Geometry: see drawing. Coordinates: mm, zero at the bounding-box minimum. A direction names the side the tool comes from. Coordinates: 2 decimals unless noted, no trailing zeros. Write each loop counter-clockwise with the first axis right and the second up, starting at its lowest first coordinate (ties: lowest second). Pieces come first, ordered by that corner, then holes.
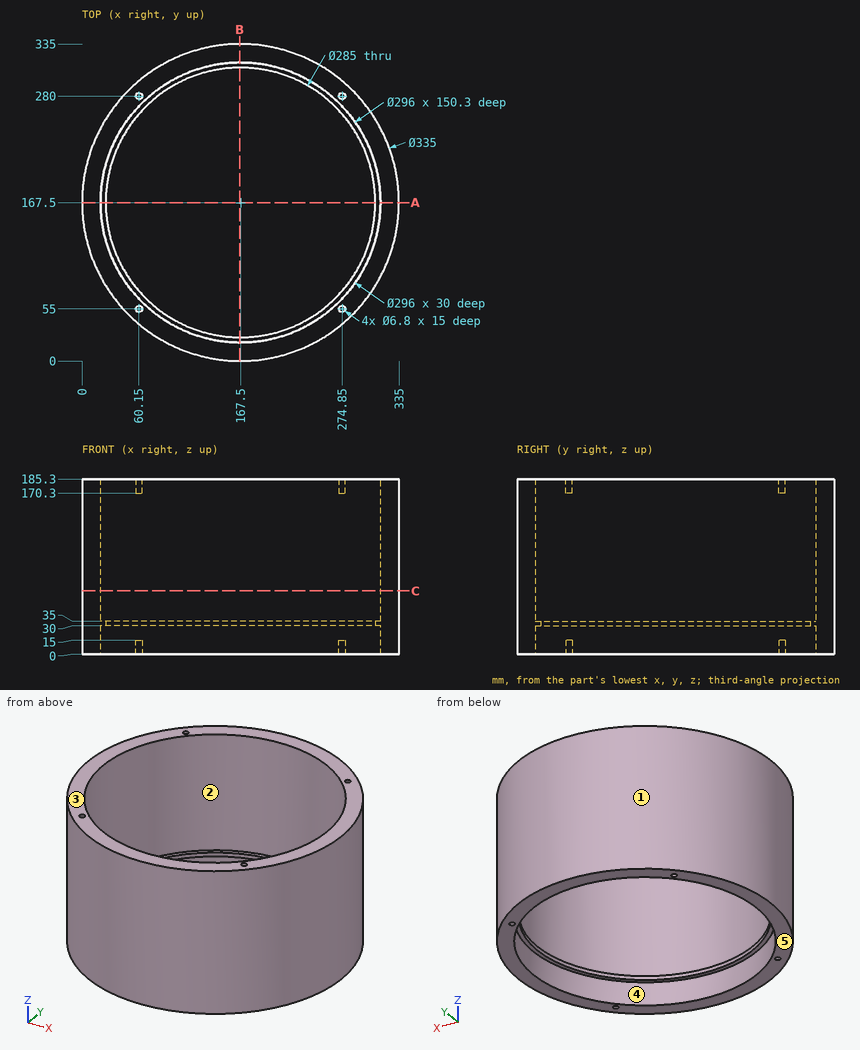
Item 1: Material intervals for probe 1 along X at (y, z) = (168.5, 40.5); probe 2 along X at (y, z) = (167, 32), sorted ascending.
Derived:
probe 1: x = 0 to 19.5, 315.5 to 335
probe 2: x = 0 to 25, 310 to 335
Item 2: Section C-C, the plane z = 67. Output: boundary loops of the cut face in (x, y).
Derived:
outline: circle Ø335 at (167.5, 167.5); hole circle Ø296 at (167.5, 167.5)
Item 3: Section A-A, the plane y = 167.5. Output: boundary loops of the cut face in (x, z), plus the area to 3 significant figures.
Derived:
outline: (0, 0) - (19.5, 0) - (19.5, 30) - (25, 30) - (25, 35) - (19.5, 35) - (19.5, 185.3) - (0, 185.3) - close; (310, 30) - (315.5, 30) - (315.5, 0) - (335, 0) - (335, 185.3) - (315.5, 185.3) - (315.5, 35) - (310, 35) - close
area: 7,280 mm2
Item 4: Pull-direction query (Y, two-part tool) for the marked faces 1, 2 and 3; classes: released by +Y, released by -Y, zero draft, split by the parting line, or undercut.
Derived:
face 1: split by the parting line
face 2: undercut
face 3: zero draft
Item 5: Pin query (flat end, axial travel): pin 1 (9 mm diameter, centred on x = 60.15, y = 280, fed in from +Z); pin 2 (1.5 mm diameter, centred on x = 130, z = 64, fed in from -Y); pin 3 (4 mm diameter, centred on x = 60.15, y = 55, fed in from +Z); pin 4 (6 mm diameter, centred on x = 274.85, y = 55, fed in from -Z). Return the tip coordinate at first contact, or that it passes through.
Derived:
pin 1: stops at z = 185.3
pin 2: stops at y = 4.08
pin 3: stops at z = 170.3
pin 4: stops at z = 15
Item 6: Set-up query: the marked faces 4 and 5. Return all of +Z, -Z, +X, -X, +Y, -Y with unobstructed straight access to the full face (end or side cutting, diameter ignored); none if empty.
Derived:
face 4: -Z
face 5: -Z, +X, -X, +Y, -Y
